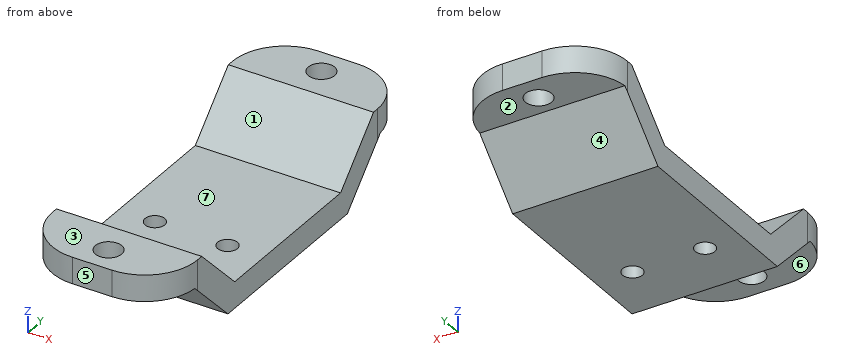
from build123d import *

# Parameters (mm, degrees)
BOSS_EXTRUDE1_DEPTH      = 8.87222
BOSS_EXTRUDE1_DEPTH_BACK = 8.87222
SKETCH2_R                = 1.6129
CUT_EXTRUDE1_DEPTH       = 10.6774
SKETCH3_R                = 1.20904
CUT_EXTRUDE2_DEPTH       = 4.2258
FILLET1_R                = 6.4516


with BuildPart() as part:
    # Sketch1 → Boss-Extrude1 (new body, two sides)
    with BuildSketch(Plane(origin=(0, 0, 0), x_dir=(0, 0, -1), z_dir=(1, 0, 0))) as boss_extrude1_sk:
        Polygon((-4.8387, 24.05126), (-1.6129, 24.05126), (-1.6129, 18.12798), (4.8387, 11.67638), (4.8387, -11.67638), (-1.6129, -18.12798), (-1.6129, -24.05126), (-4.8387, -24.05126), (-4.8387, -16.81226), (1.6129, -10.36066), (1.6129, 10.36066), (-4.8387, 16.81226), align=None)
    extrude(amount=BOSS_EXTRUDE1_DEPTH)
    extrude(boss_extrude1_sk.sketch, amount=-BOSS_EXTRUDE1_DEPTH_BACK)

    # Sketch2 → Cut-Extrude1 (cut, through all)
    with BuildSketch(Plane.XY.offset(4.8387)):
        with Locations((0, 20.82546)):
            Circle(SKETCH2_R)
    cut_extrude1 = extrude(amount=-CUT_EXTRUDE1_DEPTH, mode=Mode.SUBTRACT)

    # Mirror1: Cut-Extrude1 across plane
    add(cut_extrude1.mirror(Plane.ZX), mode=Mode.SUBTRACT)

    # Sketch3 → Cut-Extrude2 (cut, through all)
    with BuildSketch(Plane.XY.offset(-1.6129)):
        with Locations((-4.43611, -4.65328)):
            Circle(SKETCH3_R)
        with Locations((4.43611, -4.65328)):
            Circle(SKETCH3_R)
    extrude(amount=-CUT_EXTRUDE2_DEPTH, mode=Mode.SUBTRACT)

    # Fillet1
    fillet1_edges = [part.edges().sort_by_distance(p)[0] for p in [
        (-8.87222, -24.05126, 3.2258),
        (8.87222, -24.05126, 3.2258),
        (8.87222, 24.05126, 3.2258),
        (-8.87222, 24.05126, 3.2258),
    ]]
    fillet(fillet1_edges, radius=FILLET1_R)


solid = part.part
Build history of the part. All positions in model axes, mm. Face numbers are marked on the shaded views. A direction names the side the tool comes from. Give positions to 0.01 mm unless a question says otherwise; leave off trailing zeros. Order: outer loops, then holes, each group sorted by start corner. A loop starts at its lowest first (then second) coordinate and runs counter-clockwise, first axis right, second up. Notation, with made-up numbers: M -29.75,89 L -12.75,89 A28 ccw -12.75,110 Z; hole C -34,-14.75 d9. An arc over 180 degrees is marked long. Put each result on its own line as item: value.
Item 1: Slice it at C-C, the plane x = -4. Write the cut outline in (y, z).
From the geometry:
outline: M -23.85,1.61 L -18.13,1.61 L -11.68,-4.84 L -5.78,-4.84 L -5.78,-1.61 L -10.36,-1.61 L -16.81,4.84 L -23.85,4.84 Z; M -3.53,-4.84 L 11.68,-4.84 L 18.13,1.61 L 23.85,1.61 L 23.85,4.84 L 16.81,4.84 L 10.36,-1.61 L -3.53,-1.61 Z
Item 2: 3-axis set-ups, long thin cutter, end or side, ignore diameter. For the marked faces 1, 2 and 3: which of +Z, -Z, +X, -X, +Y, -Y reach the whole face in a straight line?
From the geometry:
face 1: +Z, +X, -X
face 2: -Z, +X, -X, +Y
face 3: +Z, +X, -X, +Y, -Y
Item 3: Flat gauge pins, fed straight in: pin 1 Ø1.5 at (x, y) = (-1.5, -18.5) entering from -Z; pin 2 Ø2 at (x, y) = (-4.44, -4.65) entering from +Z; pin 3 Ø1 at (x, y) = (1.5, 19) entering from -Z. Where does each tip first touch, or does it go through?
From the geometry:
pin 1: stops at z = 1.23
pin 2: passes through
pin 3: stops at z = 1.61
Item 4: Slice it at B-B, the plane z = 2.5. Write the cut outline in (x, y), plus the area to 3 significant figures.
From the geometry:
outline: M -8.87,-17.6 A6.45 ccw -2.42,-24.05 L 2.42,-24.05 A6.45 ccw 8.87,-17.6 L 8.87,-14.47 L -8.87,-14.47 Z; M -8.87,14.47 L 8.87,14.47 L 8.87,17.6 A6.45 ccw 2.42,24.05 L -2.42,24.05 A6.45 ccw -8.87,17.6 Z; hole C 0,-20.83 d3.23; hole C 0,20.83 d3.23
area: 288 mm2
Item 5: Slice it at D-D, the plane z = 0.5. Write the cut outline in (x, y), plus the area to 3 significant figures.
From the geometry:
outline: M -8.87,-17.02 L 8.87,-17.02 L 8.87,-12.47 L -8.87,-12.47 Z; M -8.87,12.47 L 8.87,12.47 L 8.87,17.02 L -8.87,17.02 Z
area: 161 mm2
Item 6: Two-plate mould, pull along Y, no slides. Class the marked faces 4, 5, 6 and 7: +Y half, -Y half, draft (parallel to the pull), parting line (faces both ways), or undercut.
From the geometry:
face 4: +Y half
face 5: -Y half
face 6: draft
face 7: undercut
Item 7: Probe line 1 (Y direction, x = 0, z = 2.5); line 2 (Y direction, x = 0, z = 3.3); line 3 (Y direction, x = -4, z = -4.5). List the from-to ranges inside material, lowest first. Write a range as [from, to].
From the geometry:
line 1: y = [-24.05, -22.44], [-19.21, -14.47], [14.47, 19.21], [22.44, 24.05]
line 2: y = [-24.05, -22.44], [-19.21, -15.27], [15.27, 19.21], [22.44, 24.05]
line 3: y = [-12.02, -5.78], [-3.53, 12.02]
Item 8: Slice it at A-A, the plane x = 0. Write the cut outline in (y, z).
From the geometry:
outline: M -24.05,1.61 L -22.44,1.61 L -22.44,4.84 L -24.05,4.84 Z; M -19.21,1.61 L -18.13,1.61 L -11.68,-4.84 L 11.68,-4.84 L 18.13,1.61 L 19.21,1.61 L 19.21,4.84 L 16.81,4.84 L 10.36,-1.61 L -10.36,-1.61 L -16.81,4.84 L -19.21,4.84 Z; M 22.44,1.61 L 24.05,1.61 L 24.05,4.84 L 22.44,4.84 Z
